Input: dimensioned drawing with shaded views. Units: mm. Origin: part minimum x, y, z. A direction names the side the tool comes from. Give positions to 0.01 mm unless a question says otherwise; leave off trailing zeros. Loops run counter-clockwise (first coordinate to the right, second up) from the corner with the lowest first, then second, coordinate; pieces in that order, holes last.
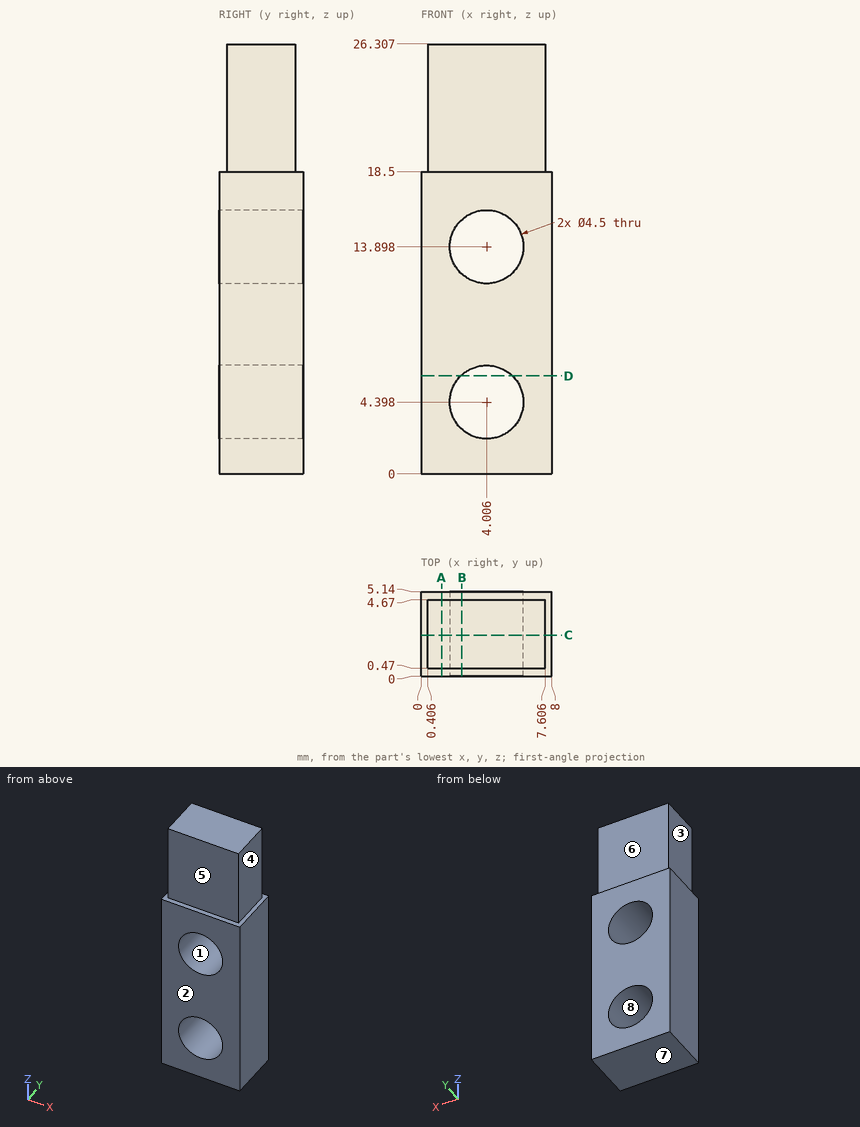
Item 1: Section query D-D on z = 6. Return loops of the section in (x, y) (1 decimal).
Values follow:
outline: (0, 0) - (2.4, 0) - (2.4, 5.1) - (0, 5.1) - close; (5.6, 0) - (8, 0) - (8, 5.1) - (5.6, 5.1) - close
Item 2: Section query C-C on y = 2.5. Return loops of the section in (x, z).
Values follow:
outline: (0, 0) - (8, 0) - (8, 18.5) - (7.61, 18.5) - (7.61, 26.31) - (0.41, 26.31) - (0.41, 18.5) - (0, 18.5) - close; hole circle Ø4.5 at (4.01, 4.4); hole circle Ø4.5 at (4.01, 13.9)
Item 3: Section query B-B on x = 2.5. Return loops of the section in (y, z).
Values follow:
outline: (0, 0) - (5.14, 0) - (5.14, 2.73) - (0, 2.73) - close; (0, 6.07) - (5.14, 6.07) - (5.14, 12.23) - (0, 12.23) - close; (0, 15.57) - (5.14, 15.57) - (5.14, 18.5) - (4.67, 18.5) - (4.67, 26.31) - (0.47, 26.31) - (0.47, 18.5) - (0, 18.5) - close
Item 4: Pin query (flat end, axial travel): pin 1 (1 mm diameter, centred on y = 2.5, z = 18.5, fed in from -X); pin 2 (2 mm diameter, centred on x = 5, z = 21.5, fed in from +Y). Return the tip coordinate at first contact, or that it passes through.
Values follow:
pin 1: stops at x = 0
pin 2: stops at y = 4.67
Item 5: Ray query, probe 1 along Z at (x, y) = (4, 0.3); probe 2 along Z at (x, y) = (3.5, 2.95) (1 decimal); probe 3 along X at (y, z) = (2, 13.75). Return the intervals inside material, ascending.
Values follow:
probe 1: z = 0 to 2.15, 6.65 to 11.65, 16.15 to 18.5
probe 2: z = 0 to 2.2, 6.6 to 11.7, 16.1 to 26.3
probe 3: x = 0 to 1.76, 6.25 to 8
Item 6: Section query A-A on x = 1.25. Return loops of the section in (y, z), plus the area to 3 significant figures.
Values follow:
outline: (0, 0) - (5.14, 0) - (5.14, 18.5) - (4.67, 18.5) - (4.67, 26.31) - (0.47, 26.31) - (0.47, 18.5) - (0, 18.5) - close
area: 128 mm2
Item 7: Draft query along X for the marked faces 1, 2 and 3. Return one class per face: +X half, -X half, draft (parallel to the pull), parting line (faces both ways), or undercut.
Values follow:
face 1: undercut
face 2: draft
face 3: -X half
Item 8: Set-up query: the marked faces 4, 5, 6, 7 and 8. Return all of +Z, -Z, +X, -X, +Y, -Y with unobstructed straight access to the full face (end or side cutting, diameter ignored); none if empty.
Values follow:
face 4: +Z, +X, +Y, -Y
face 5: +Z, +X, -X, -Y
face 6: +Z, +X, -X, +Y
face 7: -Z, +X, -X, +Y, -Y
face 8: +Y, -Y
